from build123d import *

# Parameters (mm, degrees)
PER_AGE1_D           = 5.5
PER_AGE1_DEPTH       = 35
PER_AGE1_CBORE_D     = 7.3
PER_AGE1_CBORE_DEPTH = 13
PER_AGE1_TIP         = 1.58771324


with BuildPart() as part:
    # Esquisse1 → Base-Révolution (revolve)
    with BuildSketch(Plane.XY, mode=Mode.PRIVATE) as base_r_volution_sk:
        Polygon((0, 0), (0, 6), (-8.4, 6), (-8.4, 5.75), (-9.5, 5.75), (-9.5, 6), (-63, 6), (-66, 3), (-66, 2), (-78, 2), (-78, 1.55), (-78.7, 1.55), (-78.7, 2), (-81, 2), (-81, 0), align=None)
    revolve(base_r_volution_sk.sketch.rotate(Axis((-95.795789587, 0, 0), (1, 0, 0)), 90), axis=Axis((-95.795789587, 0, 0), (1, 0, 0)))

    # Perçage1
    with Locations(Plane(origin=(0, 0, 0), x_dir=(0, 0, -1), z_dir=(1, 0, 0))):
        with Locations((0, 0)):
            CounterBoreHole(PER_AGE1_D / 2, PER_AGE1_CBORE_D / 2, PER_AGE1_CBORE_DEPTH, depth=PER_AGE1_DEPTH)
            with Locations((0, 0, -(PER_AGE1_DEPTH + PER_AGE1_TIP / 2))):  # 120° drill point
                Cone(0, PER_AGE1_D / 2, PER_AGE1_TIP, mode=Mode.SUBTRACT)


solid = part.part
Can you work these out from the model? Positions are in its coordinate system, mm. A direction names the side the tool comes from. Coordinates: 2 decimals unless noted, no trailing zeros. Order: outer loops, then holes, each group sorted by start corner. A loop starts at its lowest first (then second) coordinate and runs counter-clockwise, first axis right, second up. Notation, with made-up numbers: (45, -0.75) - (91, -0.75) arc R14 cw to (91, 19.25) - close; hole circle Ø8 at (75.5, 33). An arc over 180 degrees is marked (long way). Answer as a JSON object with one key per item and string values. Group by question number.
Q1. Imagine slicing it at A-A (x = -31). Please give me the cut outline in (y, z).
Q2. On a 3-axis mill with a long thin cutter (end or side, diameter ignored), from which of +Z, -Z, +X, -X, +Y, -Y can I reach the whole of each face in a straight line? I mean faces 4 (the face through (-72, 2, 0)), 5 (the face through (-8.96, -5.7, -0.75)), 6 (the face through (-13, 3, -1)), 7 (the face through (0, 3, -3)), 8 (the face through (-81, 0, 0)). Say none if no direction works.
Q3. I need wall thicknesses on line 1 (Y direction, x = -22.5, z = 0); line 2 (Z direction, x = -31.5, y = 1); line 3 (X direction, y = 1.25, z = 1.25). Which ranges of each line are inside material? Lowest first, please. Write a range as from..to.
Q4. Imagine slicing it at B-B (x = -64). Please give me the cut outline in (y, z).
Q5. We'd pull the mould along Y, two halves only. Please class faces 1 (the face through (-24.154, -2.685, -0.596)), 2 (the face through (-65.854, 2.791, 1.452)), 3 (the face through (-66, 2, 1)): +Y half, -Y half, draft (parallel to the pull), parting line (faces both ways), or undercut.
Q6. Will these pins go through, and if not, where does the flat tip stop? P1, Ø7, axis at y = 0, z = 0, coming from the +X side; P2, Ø1.5, axis at y = 0.5, z = 1.5, coming from the +X side; P3, Ø2, axis at y = -0.5, z = 1, coming from the +X side; P4, Ø4, axis at x = -42, y = -1.5, coming from the +Z side.
Determined:
{
 "1": {"outline": "circle Ø12 at (0, 0); hole circle Ø5.5 at (0, 0)"},
 "2": {"face 4": "-X", "face 5": "none", "face 6": "+X", "face 7": "+Z, -Z, +X, +Y, -Y", "face 8": "+Z, -Z, -X, +Y, -Y"},
 "3": {"line 1": "y = -6..-2.75, 2.75..6", "line 2": "z = -5.92..-2.56, 2.56..5.92", "line 3": "x = -81..-78.7, -78..-35.57"},
 "4": {"outline": "circle Ø10 at (0, 0)"},
 "5": {"face 1": "undercut", "face 2": "parting line", "face 3": "draft"},
 "6": {"P1": "stops at x = -13", "P2": "stops at x = -35.24", "P3": "stops at x = -35.36", "P4": "stops at z = 6"}
}
